```python
from build123d import *

# Parameters (mm, degrees)
SKETCH1_R           = 1.5
SKETCH1_R_2         = 1
BOSS_EXTRUDE1_DEPTH = 3
SKETCH2_R           = 1
BOSS_EXTRUDE2_DEPTH = 2
BOSS_EXTRUDE4_START = -3
SKETCH3_R           = 1.5
BOSS_EXTRUDE4_DEPTH = 5
SKETCH4_R           = 1.5
CUT_EXTRUDE1_DEPTH  = 168.334993352


with BuildPart() as part:
    # Sketch1 → Boss-Extrude1 (new body)
    with BuildSketch(Plane(origin=(0, 0, 0), x_dir=(1, 0, 0), z_dir=(0, 1, 0))):
        Polygon((-28, -90), (-43, -105), (-74, -115), (-74, -140), (46, -140), (46, -115), (15, -105), (0, -90), align=None)
        with Locations(Location((-28, -99, 0), (0, 0, 270))):
            Circle(SKETCH1_R, mode=Mode.SUBTRACT)
        with Locations(Location((0, -99, 0), (0, 0, 270))):
            Circle(SKETCH1_R, mode=Mode.SUBTRACT)
        with Locations(Location((-28, -109, 0), (0, 0, 270))):
            Circle(SKETCH1_R, mode=Mode.SUBTRACT)
        with Locations(Location((0, -109, 0), (0, 0, 270))):
            Circle(SKETCH1_R, mode=Mode.SUBTRACT)
        with Locations(Location((-69.77, -136, 0), (0, 0, 270))):
            Circle(SKETCH1_R_2, mode=Mode.SUBTRACT)
        with Locations(Location((-69.77, -118, 0), (0, 0, 270))):
            Circle(SKETCH1_R_2, mode=Mode.SUBTRACT)
        with Locations(Location((41.77, -136, 0), (0, 0, 90))):
            Circle(SKETCH1_R_2, mode=Mode.SUBTRACT)
        with Locations(Location((41.77, -118, 0), (0, 0, 90))):
            Circle(SKETCH1_R_2, mode=Mode.SUBTRACT)
    extrude(amount=BOSS_EXTRUDE1_DEPTH)

    # Sketch2 → Boss-Extrude2 (add)
    # profile 1 of 2: a face of its own
    with BuildSketch(Plane(origin=(0, 3, 0), x_dir=(1, 0, 0), z_dir=(0, 1, 0))):
        Polygon((-74, -115), (-74, -140), (-51, -140), (-51, -107.580645161), align=None)
        with Locations(Location((-69.77, -118, 0), (0, 0, 270))):
            Circle(SKETCH2_R, mode=Mode.SUBTRACT)
        with Locations(Location((-69.77, -136, 0), (0, 0, 270))):
            Circle(SKETCH2_R, mode=Mode.SUBTRACT)
    # profile 2 of 2: a face of its own
    with BuildSketch(Plane(origin=(0, 3, 0), x_dir=(1, 0, 0), z_dir=(0, 1, 0))):
        Polygon((46, -115), (46, -140), (23, -140), (23, -107.580645161), align=None)
        with Locations(Location((41.77, -118, 0), (0, 0, 90))):
            Circle(SKETCH2_R, mode=Mode.SUBTRACT)
        with Locations(Location((41.77, -136, 0), (0, 0, 90))):
            Circle(SKETCH2_R, mode=Mode.SUBTRACT)
    extrude(amount=BOSS_EXTRUDE2_DEPTH)

    # Sketch3 → Boss-Extrude4 (add)
    with BuildSketch(Plane(origin=(0, 3, 0), x_dir=(1, 0, 0), z_dir=(0, 1, 0)).offset(BOSS_EXTRUDE4_START)):
        Polygon((-51, -150), (23, -150), (23, -95), (5, -95), (0, -90), (-28, -90), (-33, -95), (-51, -95), align=None)
        with Locations(Location((-28, -99, 0), (0, 0, 270))):
            Circle(SKETCH3_R, mode=Mode.SUBTRACT)
        with Locations(Location((0, -99, 0), (0, 0, 270))):
            Circle(SKETCH3_R, mode=Mode.SUBTRACT)
        with Locations(Location((0, -109, 0), (0, 0, 270))):
            Circle(SKETCH3_R, mode=Mode.SUBTRACT)
        with Locations(Location((-28, -109, 0), (0, 0, 270))):
            Circle(SKETCH3_R, mode=Mode.SUBTRACT)
    extrude(amount=BOSS_EXTRUDE4_DEPTH)

    # Sketch4 → Cut-Extrude1 (cut, through all)
    with BuildSketch(Plane(origin=(0, 5, 0), x_dir=(1, 0, 0), z_dir=(0, 1, 0))):
        with Locations(Location((-46.11, -99.19, 0), (0, 0, 270))):
            Circle(SKETCH4_R)
    extrude(amount=-CUT_EXTRUDE1_DEPTH, mode=Mode.SUBTRACT)


solid = part.part
```
Source: CAD feature listing. Evaluate the final solid. Frame: model axes, mm. A direction names the side the tool comes from. Give positions to 0.01 mm unless a question says otherwise; leave off trailing zeros. Loops run counter-clockwise (first coordinate to the right, second up) from the corner with the lowest first, then second, coordinate; pieces in that order, holes last. Notation, with made-up numbers: (45, -13) -> (92, -13) arc R4 cw to (92, -7) -> close; hole circle Ø9 at (-37, -39). An arc over 180 degrees is marked (long way). Put each result on its own line as item: value. Start each with the question number.
1) Cut plane D-D (z = 109). Return loops of the section in (x, y).
2) Cut plane C-C (y = 2). State how many separate pieces and enclosed holes the cut face has, then the cut area to 3 significant figures.
3) Draft query along X for faces 4 (the face through (-74, 2, 127)), 5 (the face through (46, 2, 128)), 6 (the face through (-46.04, 2.54, 97.69)). Return one class per face: released by +X, released by -X, zero draft, split by the parting line, or undercut.
4) Cut plane B-B (z = 99). Return loops of the section in (x, y).
5) Cut plane A-A (x = -46.11). Return loops of the section in (y, z), then the cut area to 3 significant figures.
6) Material intervals for probe 1 along X at (y, z) = (3.8, 99); probe 2 along X at (y, z) = (1.15, 136); probe 3 along Z at (x, y) = (-69, 1.3), sorted ascending.
7) Reachability of faces 1 (the face through (-51, 2, 145)), 2 (the face through (23, 2, 145)), 3 (the face through (-42, 2, 95)) from +Z, -Z, +X, -X, +Y, -Y: full face, straight path, thin tool, end or side. Return the list, or none.
8) Contact query for flat-ended pins moving along their axis: P1, Ø5, axis at x = -34.5, z = 124.5, coming from the -Y side; P2, Ø2.5, axis at x = 0, z = 109, coming from the -Y side; P3, Ø1.5, axis at x = -39.5, y = 2.5, coming from the -Z side; P4, Ø1, axis at y = 3.5, z = 102.5, coming from the -X side. Output: stop coordinate, or through.
Results are:
1. outline: (-55.4, 0) -> (-29.5, 0) -> (-29.5, 5) -> (-55.4, 5) -> close; (-26.5, 0) -> (-1.5, 0) -> (-1.5, 5) -> (-26.5, 5) -> close; (1.5, 0) -> (27.4, 0) -> (27.4, 5) -> (1.5, 5) -> close
2. separate pieces: 1
2. enclosed holes: 9
2. area: 5,510 mm2
3. face 4: released by -X
3. face 5: released by +X
3. face 6: undercut
4. outline: (-51, 0) -> (-47.6, 0) -> (-47.6, 5) -> (-51, 5) -> close; (-44.62, 0) -> (-29.5, 0) -> (-29.5, 5) -> (-44.62, 5) -> close; (-26.5, 0) -> (-1.5, 0) -> (-1.5, 5) -> (-26.5, 5) -> close; (1.5, 0) -> (23, 0) -> (23, 5) -> (1.5, 5) -> close
5. outline: (0, 95) -> (5, 95) -> (5, 97.69) -> (0, 97.69) -> close; (0, 100.69) -> (5, 100.69) -> (5, 150) -> (0, 150) -> close
5. area: 260 mm2
6. probe 1: x = -51 to -47.6, -44.62 to -29.5, -26.5 to -1.5, 1.5 to 23
6. probe 2: x = -74 to -70.77, -68.77 to 40.77, 42.77 to 46
6. probe 3: z = 113.39 to 117.36, 118.64 to 135.36, 136.64 to 140
7. face 1: +Z, -X, +Y, -Y
7. face 2: +Z, +X, +Y, -Y
7. face 3: -Z, -X, +Y, -Y
8. P1: stops at y = 0
8. P2: passes through
8. P3: stops at z = 95
8. P4: stops at x = -51
